from build123d import *

# Parameters (mm, degrees)
F0_R     = 37.170022
F0_R_2   = 31.88441
F1_DEPTH = 98.552
F3_DEPTH = 51.816


with BuildPart() as f1:
    # F0 (on Top) → F1 (new body)
    with BuildSketch(Plane.XY):
        Circle(F0_R)
        Circle(F0_R_2, mode=Mode.SUBTRACT)
    extrude(amount=F1_DEPTH)

    # F2 (on face) → F3 (join)
    with BuildSketch(Plane.XY.offset(98.552)):
        with BuildLine():
            Line((-19.516608, -55.634487), (19.516608, -55.634487))
            Line((19.516608, -55.634487), (19.516608, -31.634041))
            ThreePointArc((19.516608, -31.634041), (17.761469, -32.651811), (15.953412, -33.572298))
            Line((15.953412, -33.572298), (15.953412, -52.557178))
            Line((15.953412, -52.557178), (-15.953412, -52.557178))
            Line((-15.953412, -52.557178), (-15.953412, -33.572298))
            ThreePointArc((-15.953412, -33.572298), (-17.761469, -32.651811), (-19.516608, -31.634041))
            Line((-19.516608, -31.634041), (-19.516608, -55.634487))
        make_face()
    extrude(amount=-F3_DEPTH)


solid = f1.part
Design review of the part built by this model. Coordinates are the model's own, in mm. A direction names the side the tool comes from. Give positions to 0.01 mm unless a question says otherwise; leave off trailing zeros. Write each loop counter-clockwise with the first axis right and the second up, starting at its lowest first coordinate (ties: lowest second). Pieces come first, ordered by that corner, then holes. Notation, with made-up numbers: M 6.5,13.5 L 63.5,13.5 A34 ccw 63.5,46.5 Z; hole C -33,47.5 d4. An arc over 180 degrees is marked long. Answer as a JSON object with one key per item and string values. Group by question number.
1) Clearance check with flat-ended pins moving along their axes: pin 1 Ø6 at (y, z) = (-23, 30.5) entering from +X; pin 2 Ø5.5 at (y, z) = (-39.5, 80.5) entering from -X; pin 3 Ø2 at (x, z) = (19.5, 66.5) entering from +Y; pin 4 Ø4 at (y, z) = (2, 50) entering from -X. State where each tip first meets the part, or that it passes through.
2) We need section A-A (x = 0). Give the boundary of the cut face in (y, z).
3) We need section D-D (y = 0). Give the boundary of the cut face in (x, z).
4) We need section B-B (z = 91.5). Give the boundary of the cut face in (x, y).
5) For line 1 along Y through (x, z) = (-2, 93); line 2 along Y through (x, z) = (10, 76); line 3 along X through (y, z) = (-39.5, 78), list the stretches that pass through material, from the lowest coordinate up.
6) Tool access review of faces 1 (the face through (19.517, -44, 73)), 2 (the face through (15.953, -43, 73)), 3 (the face through (-19.517, -43, 73)): name each direction out of +Z, -Z, +X, -X, +Y, -Y from which nothing blocks a thin tool from reaching the whole face with its end or side.
7) Mouldability with a two-part tool opening along Y and no side actions: class faces 4 (the face through (-15.953, -43, 73)), 5 (the face through (16, 28, 0)), 6 (the face through (0, -55.634, 73)) as released by +Y, released by -Y, zero draft, split by the parting line, or undercut.
8) We need section C-C (y = -49). Give the boundary of the cut face in (x, z).
Answer key:
{
 "1": {"pin 1": "stops at x = 31.33", "pin 2": "stops at x = -19.52", "pin 3": "stops at y = 32.24", "pin 4": "stops at x = -37.17"},
 "2": {"outline": "M -55.63,46.74 L -52.56,46.74 L -52.56,98.55 L -55.63,98.55 Z; M -37.17,0 L -31.88,0 L -31.88,98.55 L -37.17,98.55 Z; M 31.88,0 L 37.17,0 L 37.17,98.55 L 31.88,98.55 Z"},
 "3": {"outline": "M -37.17,0 L -31.88,0 L -31.88,98.55 L -37.17,98.55 Z; M 31.88,0 L 37.17,0 L 37.17,98.55 L 31.88,98.55 Z"},
 "4": {"outline": "M -19.52,-55.63 L 19.52,-55.63 L 19.52,-31.63 A37.17 ccw long -19.52,-31.63 Z; hole C 0,0 d63.77; hole M -15.95,-52.56 L 15.95,-52.56 L 15.95,-33.57 A37.17 cw -15.95,-33.57 Z"},
 "5": {"line 1": "y = -55.63 to -52.56, -37.12 to -31.82, 31.82 to 37.12", "line 2": "y = -55.63 to -52.56, -35.8 to -30.28, 30.28 to 35.8", "line 3": "x = -19.52 to -15.95, 15.95 to 19.52"},
 "6": {"face 1": "+Z, -Z, +X, -Y", "face 2": "+Z, -Z", "face 3": "+Z, -Z, -X, -Y"},
 "7": {"face 4": "undercut", "face 5": "zero draft", "face 6": "released by -Y"},
 "8": {"outline": "M -19.52,46.74 L -15.95,46.74 L -15.95,98.55 L -19.52,98.55 Z; M 15.95,46.74 L 19.52,46.74 L 19.52,98.55 L 15.95,98.55 Z"}
}
